```python
from build123d import *

# Parameters (mm, degrees)
SKETCH_2_W             = 26
SKETCH_2_H             = 38
SKETCH_2_R             = 1.8
SKETCH_2_R_2           = 5
EXTRUDE_1_DEPTH        = 4
EXTRUDE_START          = -25
SKETCH_3_R             = 4
SKETCH_3_R_2           = 1.55
EXTRUDE_2_DEPTH        = 3.6
FILLET_1_R             = 2
RIB_1_REACH            = 48.579
SKETCH_4_WALL_W        = 112.976143744
SKETCH_4_WALL_H        = 2
PATTERN_LINEAR_1_COUNT = 4
PATTERN_LINEAR_1_PITCH = 6
CHAMFER_1_SIZE         = 0.8


with BuildPart() as part:
    # 草图2 → 凸台-拉伸1 (new body)
    with BuildSketch(Plane(origin=(0, 0, 0), x_dir=(1, 0, 0), z_dir=(0, 1, 0))):
        with Locations((0, 6)):
            Rectangle(SKETCH_2_W, SKETCH_2_H)
        with Locations(Location((-8.131727984, 8.131727984, 0), (0, 0, 270))):
            Circle(SKETCH_2_R, mode=Mode.SUBTRACT)
        with Locations(Location((8.131727984, 8.131727984, 0), (0, 0, 270))):
            Circle(SKETCH_2_R, mode=Mode.SUBTRACT)
        with Locations(Location((8.131727984, -8.131727984, 0), (0, 0, 270))):
            Circle(SKETCH_2_R, mode=Mode.SUBTRACT)
        with Locations(Location((-8.131727984, -8.131727984, 0), (0, 0, 270))):
            Circle(SKETCH_2_R, mode=Mode.SUBTRACT)
        with Locations(Location((0, 0, 0), (0, 0, 270))):
            Circle(SKETCH_2_R_2, mode=Mode.SUBTRACT)
    extrude(amount=EXTRUDE_1_DEPTH)

    # 草图3 → 凸台-拉伸2 (add)
    with BuildSketch(Plane.XY.offset(EXTRUDE_START)):
        with BuildLine():
            Line((-13, 20), (-13, 4))
            Line((-13, 4), (13, 4))
            Line((13, 4), (13, 20))
            ThreePointArc((13, 20), (0, 33), (-13, 20))
        make_face()
        with Locations((0, 20)):
            Circle(SKETCH_3_R, mode=Mode.SUBTRACT)
        with Locations((-1.621876461, 28.343831059)):
            Circle(SKETCH_3_R_2, mode=Mode.SUBTRACT)
        with Locations((8.343831059, 21.621876461)):
            Circle(SKETCH_3_R_2, mode=Mode.SUBTRACT)
        with Locations((1.621876461, 11.656168941)):
            Circle(SKETCH_3_R_2, mode=Mode.SUBTRACT)
        with Locations((-8.343831059, 18.378123539)):
            Circle(SKETCH_3_R_2, mode=Mode.SUBTRACT)
    extrude(amount=EXTRUDE_2_DEPTH)

    # 圆角1
    fillet_1_edges = [part.edges().sort_by_distance(p)[0] for p in [
        (0, 4, -21.4),
        (0, 0, -25),
        (13, 2, 13),
        (-13, 2, 13),
    ]]
    fillet(fillet_1_edges, radius=FILLET_1_R)

    # 草图4 wall → 筋1 (add, up to next)
    with BuildSketch(Plane(origin=(-8.343831059, 6.7, -18.7), x_dir=(0, -0.707106781187, 0.707106781187), z_dir=(0, 0.707106781187, 0.707106781187)), mode=Mode.PRIVATE) as rib_1_sk1:
        Rectangle(SKETCH_4_WALL_W, SKETCH_4_WALL_H)
    rib_1_tool1 = extrude(rib_1_sk1.sketch, amount=-RIB_1_REACH, mode=Mode.PRIVATE) - part.part
    rib_1 = rib_1_tool1.solids().sort_by_distance((-8.343831059, 6.7, -18.7))[0]
    add(rib_1)

    # 阵列(线性)1: 筋1 ×4
    with Locations(*[(i * PATTERN_LINEAR_1_PITCH, 0, 0) for i in range(1, PATTERN_LINEAR_1_COUNT)]):
        add(rib_1)

    # 倒角1
    chamfer_1_edges = [part.edges().sort_by_distance(p)[0] for p in [
        (6.793831059, 21.621876461, -21.4),
        (0.071876461, 11.656168941, -21.4),
        (-3.171876461, 28.343831059, -21.4),
        (-9.893831059, 18.378123539, -21.4),
    ]]
    chamfer(chamfer_1_edges, length=CHAMFER_1_SIZE)


solid = part.part
```
Source: CAD feature listing. Evaluate the final solid. Frame: model axes, mm. A direction names the side the tool comes from. Give positions to 0.01 mm unless a question says otherwise; leave off trailing zeros. Loops run counter-clockwise (first coordinate to the right, second up) from the corner with the lowest first, then second, coordinate; pieces in that order, holes last. Notation, with made-up numbers: (2.25, -5) -> (57.25, -5) arc R34 ccw to (57.25, 25) -> close; hole circle Ø11 at (-34, 10.5). An arc over 180 degrees is marked (long way). Use a Markdown table: item, result. Add a question column.
(1) Section query B-B (x = 7.25). Count the separate pieces of the cut face and the enclosed holes in it, then the cut area to 3 significant figures.
(2) First-contact query: pin 1 Ø2.5 at (y, z) = (7.5, -19) entering from -X; pin 2 Ø3 at (x, y) = (4.5, 18) entering from +Z; pin 3 Ø1.6 at (y, z) = (5.5, -18.5) entering from +X. Flat tips, straight axial feed; report the tip coordinate or a pass-through.
(3) Section query C-C (z = -12.5). Output: boundary loops of the cut face in (x, y).
(4) Pull-direction query (Z, two-part tool) for faces 1 (the face through (-4.88, 1.97, -1.08)), 2 (the face through (-2, 7, -19)), 3 (the face through (-9.57, 17.43, -23.62)); classes: +Z half, -Z half, draft (parallel to the pull), parting line (faces both ways), or undercut.
(5) Ray query, line 1 (Y direction, x = 0, z = -23.1); line 2 (Y direction, x = -2, z = -23); line 3 (X direction, y = 3.2, z = 0). Return the intervals inside material, ascending.
(6) Access query for faces 4 (the face through (4, 7, -19)), 5 (the face through (-1.344, 6, -20)), 6 (the face through (10.656, 6, -20)). Directions: +Z, -Z, +X, -X, +Y, -Y. A direction counts if a zero-diameter tool reaches every point of the face in a straight line with its end or side. Return the directions, or none.
(7) Section query A-A (z = 0). Output: boundary loops of the cut face in (x, y).
Checked values:
| question | item | result |
|---|---|---|
| 1 | separate pieces | 4 |
| 1 | enclosed holes | 0 |
| 1 | area | 215 mm^2 |
| 2 | pin 1 | x = -9.34 |
| 2 | pin 2 | z = -21.4 |
| 2 | pin 3 | x = 10.66 |
| 3 | outline | (-13, 0) -> (13, 0) -> (13, 4) -> (-13, 4) -> close |
| 4 | face 1 | undercut |
| 4 | face 2 | +Z half |
| 4 | face 3 | draft |
| 5 | line 1 | 0 to 16, 24 to 33 |
| 5 | line 2 | 0 to 16.54, 23.46 to 26.84, 29.85 to 32.85 |
| 5 | line 3 | -13 to -5, 5 to 13 |
| 6 | face 4 | +Z, +X, -X, +Y |
| 6 | face 5 | +Z, +Y |
| 6 | face 6 | +Z, +X, +Y |
| 7 | outline | (-13, 0) -> (-5, 0) -> (-5, 4) -> (-13, 4) -> close; (5, 0) -> (13, 0) -> (13, 4) -> (5, 4) -> close |
